```python
from build123d import *

# Parameters (mm, degrees)
F0_R     = 44.45
F0_R_2   = 1.5875
F1_DEPTH = 3.175


# Not quite as in the source:
# - a length typed as a fraction of an inch, garbled in the dataset ("3 / 203.2 mm" for 3/8 in), is restored


with BuildPart() as f1:
    # F0 (on Top) → F1 (new body)
    with BuildSketch(Plane.XY):
        Circle(F0_R)
        with BuildLine():
            ThreePointArc((40.4610120981, 3.81), (40.5952283629, 1.9071009851), (40.64, 0))
            ThreePointArc((40.64, 0), (40.5952283629, -1.9071009851), (40.4610120981, -3.81))
            ThreePointArc((40.4610120981, -3.81), (28.7368195874, -28.7368195874), (3.81, -40.4610120981))
            ThreePointArc((3.81, -40.4610120981), (0, -40.64), (-3.81, -40.4610120981))
            ThreePointArc((-3.81, -40.4610120981), (-28.7368195874, -28.7368195874), (-40.4610120981, -3.81))
            ThreePointArc((-40.4610120981, -3.81), (-40.64, 0), (-40.4610120981, 3.81))
            ThreePointArc((-40.4610120981, 3.81), (-28.7368195874, 28.7368195874), (-3.81, 40.4610120981))
            ThreePointArc((-3.81, 40.4610120981), (0, 40.64), (3.81, 40.4610120981))
            ThreePointArc((3.81, 40.4610120981), (28.7368195874, 28.7368195874), (40.4610120981, 3.81))
        make_face(mode=Mode.SUBTRACT)
        with BuildLine():
            ThreePointArc((40.4610120981, -3.81), (40.5952283629, -1.9071009851), (40.64, 0))
            ThreePointArc((40.64, 0), (40.5952283629, 1.9071009851), (40.4610120981, 3.81))
            Line((40.4610120981, 3.81), (3.81, 3.81))
            Line((3.81, 3.81), (3.81, 0))
            Line((3.81, 0), (3.81, -3.81))
            Line((3.81, -3.81), (40.4610120981, -3.81))
        make_face()
        with BuildLine():
            Line((3.81, 3.81), (3.81, 40.4610120981))
            ThreePointArc((3.81, 40.4610120981), (0, 40.64), (-3.81, 40.4610120981))
            Line((-3.81, 40.4610120981), (-3.81, 3.81))
            Line((-3.81, 3.81), (0, 3.81))
            Line((0, 3.81), (3.81, 3.81))
        make_face()
        Polygon((3.81, 0), (3.81, 3.81), (0, 3.81), (-3.81, 3.81), (-3.81, 0), (-3.81, -3.81), (0, -3.81), (3.81, -3.81), align=None)
        Circle(F0_R_2, mode=Mode.SUBTRACT)
        with BuildLine():
            ThreePointArc((-3.81, -40.4610120981), (0, -40.64), (3.81, -40.4610120981))
            Line((3.81, -40.4610120981), (3.81, -3.81))
            Line((3.81, -3.81), (0, -3.81))
            Line((0, -3.81), (-3.81, -3.81))
            Line((-3.81, -3.81), (-3.81, -40.4610120981))
        make_face()
        with BuildLine():
            Line((-3.81, 3.81), (-40.4610120981, 3.81))
            ThreePointArc((-40.4610120981, 3.81), (-40.64, 0), (-40.4610120981, -3.81))
            Line((-40.4610120981, -3.81), (-3.81, -3.81))
            Line((-3.81, -3.81), (-3.81, 0))
            Line((-3.81, 0), (-3.81, 3.81))
        make_face()
    extrude(amount=F1_DEPTH)


solid = f1.part
```
Source: CAD feature listing. Evaluate the final solid. Frame: model axes, mm. A direction names the side the tool comes from. Give positions to 0.01 mm unless a question says otherwise; leave off trailing zeros. Loops run counter-clockwise (first coordinate to the right, second up) from the corner with the lowest first, then second, coordinate; pieces in that order, holes last. Notation, with made-up numbers: M -16,-19.75 L -11,-19.75 A10 ccw -11,-14.75 Z; hole C 9.5,77.5 d11. An arc over 180 degrees is marked long. Put each result on its own line as item: value.
Q1. Line query: probe 1 along Y at (x, z) = (0, 1.2); probe 2 along X at (y, z) = (15, 2.8); probe 3 along Y at (x, z) = (-19, 0.2). Output: solid intervals per line, ascending. Write a range as [from, to].
Response values:
probe 1: y = [-44.45, -1.59], [1.59, 44.45]
probe 2: x = [-41.84, -37.77], [-3.81, 3.81], [37.77, 41.84]
probe 3: y = [-40.18, -35.93], [-3.81, 3.81], [35.93, 40.18]
Q2. Mould query, pull axis X, two halves, no side actions, for faces 1 (the flat face through (22, -3.81, 2)), 2 (the cylindrical face through (42.397, 13.352, 1.565)), 3 (the flat face through (-4, 0, 0)). Classes: released by +X, released by -X, zero draft, split by the parting line, or undercut.
Response values:
face 1: undercut
face 2: split by the parting line
face 3: zero draft
Q3. Section D-D (x = 24.5). Return the cut outline in (y, z) (3 decimals).
Response values:
outline: M -37.088,0 L -32.425,0 L -32.425,3.175 L -37.088,3.175 Z; M -3.81,0 L 3.81,0 L 3.81,3.175 L -3.81,3.175 Z; M 32.425,0 L 37.088,0 L 37.088,3.175 L 32.425,3.175 Z
Q4. Section B-B (z = 2.05). Count the separate pieces of the cut face and the enclosed holes in it, and give its area (3 significant figures).
Response values:
separate pieces: 1
enclosed holes: 5
area: 2,190 mm²
Q5. Reachability of faces 4 (the flat face through (-4, 0, 3.175)), 5 (the flat face through (22, 3.81, 2)) from +Z, -Z, +X, -X, +Y, -Y: full face, straight path, thin tool, end or side. Return the list, or none.
Response values:
face 4: +Z, +X, -X, +Y, -Y
face 5: +Z, -Z
Q6. Pin query (flat end, axial travel): P1, Ø1.9, axis at x = 0, y = 0, coming from the -Z side; P2, Ø1.6, axis at y = -17, z = 2, coming from the +X side; P3, Ø1, axis at x = 22, z = 1, coming from the -Y side; P4, Ø1.5, axis at x = -9, z = 0.5, coming from the +Y side. Return the tip coordinate at first contact, or that it passes through.
Response values:
P1: passes through
P2: stops at x = 41.39
P3: stops at y = -38.9
P4: stops at y = 43.68
